```python
from build123d import *

# Parameters (mm, degrees)
SKETCH1_R           = 2.5
BOSS_EXTRUDE1_DEPTH = 1.5
CIRPATTERN1_COUNT   = 2
CIRPATTERN1_ANGLE   = 90
FILLET1_R           = 2
SKETCH3_R           = 2.5
CUT_EXTRUDE2_DEPTH  = 0.75
CUT_EXTRUDE2_DRAFT  = -60


with BuildPart() as part:
    # Sketch1 → Boss-Extrude1 (new body)
    with BuildSketch(Plane(origin=(0, 0, 0), x_dir=(1, 0, 0), z_dir=(0, 1, 0))):
        with BuildLine():
            Line((-7.5, 0), (7.5, 0))
            Line((7.5, 0), (7.5, 12.5))
            ThreePointArc((7.5, 12.5), (0, 20), (-7.5, 12.5))
            Line((-7.5, 12.5), (-7.5, 0))
        make_face()
        with Locations(Location((0, 12, 0), (0, 0, 270))):
            Circle(SKETCH1_R, mode=Mode.SUBTRACT)
    boss_extrude1 = extrude(amount=BOSS_EXTRUDE1_DEPTH)

    # CirPattern1: Boss-Extrude1 ×2 about axis
    cirpattern1_axis = Axis((-7.5, 1.5, 0), (-1, 0, 0))
    for i in range(1, CIRPATTERN1_COUNT):
        add(boss_extrude1.rotate(cirpattern1_axis, i * CIRPATTERN1_ANGLE / (CIRPATTERN1_COUNT - 1)))

    # Fillet1
    fillet1_edges = [part.edges().sort_by_distance(p)[0] for p in [
        (0, 1.5, 1.5),
        (0, 0, 0),
    ]]
    fillet(fillet1_edges, radius=FILLET1_R)


with BuildPart() as cut_extrude2_tool:
    # Sketch3 → Cut-Extrude2 (with draft: the straight prism first)
    with BuildSketch(Plane(origin=(0, 0.75, 0), x_dir=(-1, 0, 0), z_dir=(0, -1, 0))):
        with Locations(Location((0, 12, 0), (0, 0, 90))):
            Circle(SKETCH3_R)
    extrude(amount=CUT_EXTRUDE2_DEPTH)
    # Cut-Extrude2: the draft: its side faces are tilted about the plane it starts from
    cut_extrude2_sides = [cut_extrude2_tool.faces().sort_by_distance(p)[0] for p in [
        (0, 0.375, -9.5),
    ]]
    draft(cut_extrude2_sides, Plane(origin=(0, 0.75, 0), x_dir=(-1, 0, 0), z_dir=(0, -1, 0)), CUT_EXTRUDE2_DRAFT)


with BuildPart() as part_1:
    add(part.part)

    # Cut-Extrude2: cut by cut_extrude2_tool
    add(cut_extrude2_tool.part, mode=Mode.SUBTRACT)


solid = part_1.part
```
Could you check a few things on this model? Use its own coordinates, in mm. A direction names the side the tool comes from. Round coordinates to 2 decimals unless told otherwise and drop trailing zeros. Write each loop counter-clockwise with the first axis right and the second up, starting at its lowest first coordinate (ties: lowest second). Pieces come first, ordered by that corner, then holes.
(1) Suppose I cut it at D-D on y = -4.5. Write out the boundary of the cut face in (x, z).
Findings below:
outline: (-7.5, 0) - (7.5, 0) - (7.5, 1.5) - (-7.5, 1.5) - close
(2) Which directions (+Z, -Z, +X, -X, +Y, -Y) give clear straight access to the entire face, cutting with the end or side of a thin tool? Please do faces 5 (the face through (-1.8, -8.5, 0)), 6 (the face through (0, 1.5, -8)).
Findings below:
face 5: -Z, +X, -X, -Y
face 6: +Z, -Z, +X, -X, +Y
(3) Suppose I cut it at B-B on x = 0. Write out the boundary of the cut face in (y, z).
Findings below:
outline: (-18.5, 0) - (-13, 0) - (-13, 1.5) - (-18.5, 1.5) - close; (-8, 0) - (-2, 0) arc R2 cw to (0, -2) - (0, -8.2) - (0.75, -9.5) - (1.5, -9.5) - (1.5, -0.5) arc R2 ccw to (-0.5, 1.5) - (-8, 1.5) - close; (0, -20) - (1.5, -20) - (1.5, -14.5) - (0.75, -14.5) - (0, -15.8) - close
(4) Suppose I cut it at A-A on y = -10.5. Write out the boundary of the cut face in (x, z), and give its area (3 significant figures).
Findings below:
outline: (-7.5, 0) - (-2.5, 0) - (-2.5, 1.5) - (-7.5, 1.5) - close; (2.5, 0) - (7.5, 0) - (7.5, 1.5) - (2.5, 1.5) - close
area: 15.0 mm2
(5) Suppose I cut it at C-C on z = -12. Write out the boundary of the cut face in (x, y).
Findings below:
outline: (-7.5, 0) - (-3.8, 0) - (-2.5, 0.75) - (-2.5, 1.5) - (-7.5, 1.5) - close; (2.5, 0.75) - (3.8, 0) - (7.5, 0) - (7.5, 1.5) - (2.5, 1.5) - close
(6) Thinking about a two-plate mould opening in X: for faces 1 (the face through (0, -13, 1)), 2 (the face through (-0.1, -7.6, 1.5)), 3 (the face through (-7.5, 0.3, -2.9)), 4 (the face through (0.1, 1.1, -14.5)), which applies, +X half, -X half, draft (parallel to the pull), parting line (faces both ways), or undercut?
Findings below:
face 1: undercut
face 2: draft
face 3: -X half
face 4: undercut
(7) For pin 1 (1 mm diameter, centred on x = -3.5, z = -4.5, fed in from -Y); pin 2 (3 mm diameter, centred on x = 0, z = -12, fed in from +Y); pin 3 (4.5 mm diameter, centred on x = 3, y = -12.5, fed in from -Z), each with a flat end and sliding along its axis, tell me the tip position at first contact or that it passes through.
Findings below:
pin 1: stops at y = 0
pin 2: passes through
pin 3: stops at z = 0
(8) If I drill on probe 1 along X at (y, z) = (-10.5, 0.65); probe 2 along Z at (x, y) = (-5.75, -5), over which ranges is the centre line in solid material (lowest first)?
Findings below:
probe 1: x = -7.5 to -2.5, 2.5 to 7.5
probe 2: z = 0 to 1.5
